Could you check a few things on this model? Use its own coordinates, in mm. Coordinates: 2 decimals unless noted, no trailing zeros. Loops run counter-clockwise (first coordinate to the right, second up) from the corner with the lowest first, then second, coordinate; pieces in that order, holes last.
1) Imagine slicing it at A-A on y = 0. Please give me the cut outline in (x, z) (3 decimals), plus the area to 3 significant figures.
2) If I drill on line 1 along Z through (x, y) = (-3, -0.15); line 2 along X through (y, z) = (0.1, -25); line 3 along X through (y, z) = (-0.6, -20), over which ranges is the centre line in solid material (lowest first)?
3) Imagine slicing it at B-B on z = -20. Please give me the cut outline in (x, y), plus the area to 3 significant figures.
4) Thinking about a two-plate mould opening in Z: for faces 1 (the face through (24.19, -0.38, -14.77)), 2 (the face through (-24.19, -0.38, -14.77)), which applies, released by +Z, released by -Z, zero draft, split by the parting line, or undercut?
5) Imagine slicing it at C-C on x = 5. Please give me the cut outline in (y, z).
```python
from build123d import *

# Parameters (mm, degrees)
SWEEP3_PROFILE_R = 1.27


with BuildPart() as part:
    # Sweep3: sweep along a path in Sketch1
    with BuildLine(Plane(origin=(0, 0, 0), x_dir=(1, 0, 0), z_dir=(0, 1, 0))) as sweep3_path:
        Line((0, 0), (-22.225, 0))
        ThreePointArc((-22.225, 0), (-24.47006403, 0.92993597), (-25.4, 3.175))
        Line((-25.4, 3.175), (-25.4, 26.035))
        ThreePointArc((-25.4, 26.035), (-24.47006403, 28.28006403), (-22.225, 29.21))
        Line((-22.225, 29.21), (0, 29.21))
    # Sweep3 profile (on start of the path) → Sweep3 (sweep)
    with BuildSketch(Plane(origin=(0, 0, 0), x_dir=(0, 0, -1), z_dir=(-1, 0, 0))):
        Circle(SWEEP3_PROFILE_R)
    sweep3 = sweep(path=sweep3_path.line)

    # Mirror1: Sweep3 across plane
    add(sweep3.mirror(Plane(origin=(0, 0, 0), x_dir=(0, 0, 1), z_dir=(1, 0, 0))))


solid = part.part
```
Filled in:
1. outline: (-26.67, -26.035) arc R4.445 ccw to (-22.225, -30.48) - (22.225, -30.48) arc R4.445 ccw to (26.67, -26.035) - (26.67, -3.175) arc R4.445 ccw to (22.225, 1.27) - (-22.225, 1.27) arc R4.445 ccw to (-26.67, -3.175) - close; hole (-24.13, -26.035) arc R1.905 ccw to (-22.225, -27.94) - (22.225, -27.94) arc R1.905 ccw to (24.13, -26.035) - (24.13, -3.175) arc R1.905 ccw to (22.225, -1.27) - (-22.225, -1.27) arc R1.905 ccw to (-24.13, -3.175) - close
1. area: 393 mm2
2. line 1: z = -30.47 to -27.95, -1.26 to 1.26
2. line 2: x = -26.67 to -24.13, 24.13 to 26.67
2. line 3: x = -26.52 to -24.28, 24.28 to 26.52
3. outline: circle Ø2.54 at (-25.4, 0); circle Ø2.54 at (25.4, 0)
3. area: 10.1 mm2
4. face 1: undercut
4. face 2: undercut
5. outline: circle Ø2.54 at (0, -29.21); circle Ø2.54 at (0, 0)
